Design review of the part built by this model. Coordinates are the model's own, in mm. A direction names the side the tool comes from. Round coordinates to 2 decimals unless told otherwise and drop trailing zeros. Order: outer loops, then holes, each group sorted by start corner. A loop starts at its lowest first (then second) coordinate and runs counter-clockwise, first axis right, second up. Notation, with made-up numbers: M 42.5,-19 L 63.5,-19 A19 cw 63.5,-9 Z; hole C 85,-2.5 d11. An arc over 180 degrees is marked long. Use a Markdown table: item, result. Add a question column.
(1) Take a section at A-A (x = 678.5). Write out the cut boundary in (y, z), then the cut area to 3 significant figures.
(2) The part is to be moulded in two halves that separate along Z. For faces 1 (the face through (832.295, -1.69, 56.85)), 2 (the face through (752, 0, 34)), 3 (the face through (872.457, -1.69, 133.828)), say which applies: released by +Z, released by -Z, zero draft, split by the parting line, or undercut.
(3) For pin 1 (1 mm diameter, centred on y = -1.5, z = 42, fed in from +X); pin 2 (1.7 mm diameter, centred on x = 860.5, y = -1, fed in from -Z); pin 3 (1 mm diameter, centred on y = -1.5, z = 155, fed in from +X); pin 4 (8 mm diameter, centred on x = 598, z = 165, fed in from +Y), all flat-tipped, find the tip position at first contact; note any pin that passes through.
(4) To check wall thickness, follow probe 1 along Z at (x, y) = (849.5, -2.2); probe 2 along Z at (x, y) = (784, -0.8); probe 3 along Z at (x, y) = (637, -1.9). State the ranges of each line that lie inside material, in increasing order. Write a range as from..to.
(5) Take a section at B-B (x = 827). Write out the cut boundary in (y, z), then the cut area to 3 significant figures.
(6) Take a section at C-C (z = 121). Write out the cut boundary in (x, y).
(7) Machinability: for faces 4 (the face through (831.6, -1.7, 141.3)), 5 (the face through (752, -3.429, 34)), which of the approach directions +Z, -Z, +X, -X, +Y, -Y give a long, thin tool a straight path to every point of the face, cutting with its end or side? Answer none if there is none.
(8) Take a section at D-D (z = 78). Write out the cut boundary in (x, y), then the cut area to 3 significant figures.
```python
from build123d import *

# Parameters (mm, degrees)
F0_W     = 3.81
F0_H     = 19.05
F1_DEPTH = 3.429


# Not quite as in the source:
# - ends of sketch curves that miss each other by under 0.0002 mm in the source are joined


with BuildPart() as f1:
    # F0 (on Front) → F1 (new body)
    with BuildSketch(Plane.XZ):
        with BuildLine():
            Line((641.7700144, 153.9733014), (749.7200144, 153.9733014))
            Line((749.7200144, 153.9733014), (749.7200144, 157.1483014))
            Line((749.7200144, 157.1483014), (768.7700144, 157.1483014))
            Line((768.7700144, 157.1483014), (768.7700144, 153.9733014))
            Line((768.7700144, 153.9733014), (800.5200144, 153.9733014))
            ThreePointArc((800.5200144, 153.9733014), (831.9509108237, 140.9541978237), (844.9700144, 109.5233014))
            Line((844.9700144, 109.5233014), (844.9700144, 87.9333014))
            ThreePointArc((844.9700144, 87.9333014), (831.9509108237, 56.5024049763), (800.5200144, 43.4833014))
            Line((800.5200144, 43.4833014), (768.7700144, 43.4833014))
            Line((768.7700144, 43.4833014), (768.7700144, 40.3083014))
            Line((768.7700144, 40.3083014), (749.7200144, 40.3083014))
            Line((749.7200144, 40.3083014), (749.7200144, 43.4833014))
            Line((749.7200144, 43.4833014), (641.7700144, 43.4833014))
            Line((641.7700144, 43.4833014), (641.7700144, 40.3083014))
            Line((641.7700144, 40.3083014), (622.7200144, 40.3083014))
            Line((622.7200144, 40.3083014), (622.7200144, 43.4833014))
            Line((622.7200144, 43.4833014), (559.2200144, 43.4833014))
            Line((559.2200144, 43.4833014), (559.2200144, 33.9583014))
            Line((559.2200144, 33.9583014), (623.5700762, 10.5367836))
            ThreePointArc((623.5700762, 10.5367836), (630.9394695232, 8.4681877562), (638.536009535, 7.5302985912))
            Line((638.536009535, 7.5302985912), (814.9544788, -0.844042))
            ThreePointArc((814.9544788, -0.844042), (848.1989075574, 9.5280670864), (866.95206277, 38.8724395401))
            Line((866.95206277, 38.8724395401), (877.8095982, 87.7019074))
            ThreePointArc((877.8095982, 87.7019074), (879.0206956, 98.7282890028), (877.80959757, 109.7546698599))
            Line((877.80959757, 109.7546698599), (866.9520634, 158.5841634))
            ThreePointArc((866.9520634, 158.5841634), (848.1988981839, 187.9285174732), (814.954479338, 198.3006334659))
            Line((814.954479338, 198.3006334659), (638.5360102, 189.9262902))
            ThreePointArc((638.5360102, 189.9262902), (630.9394701135, 188.9883897624), (623.5700733762, 186.9198015582))
            Line((623.5700733762, 186.9198015582), (559.2200144, 163.4983014))
            Line((559.2200144, 163.4983014), (559.2200144, 153.9733014))
            Line((559.2200144, 153.9733014), (622.7200144, 153.9733014))
            Line((622.7200144, 153.9733014), (622.7200144, 157.1483014))
            Line((622.7200144, 157.1483014), (641.7700144, 157.1483014))
            Line((641.7700144, 157.1483014), (641.7700144, 153.9733014))
        make_face()
        with Locations((860.8450144, 98.7283014)):
            Rectangle(F0_W, F0_H, mode=Mode.SUBTRACT)
    extrude(amount=F1_DEPTH)


solid = f1.part
```
Verdict:
| question | item | result |
|---|---|---|
| 1 | outline | M -3.43,5.63 L 0,5.63 L 0,43.48 L -3.43,43.48 Z; M -3.43,153.97 L 0,153.97 L 0,191.82 L -3.43,191.82 Z |
| 1 | area | 260 mm^2 |
| 2 | face 1 | undercut |
| 2 | face 2 | zero draft |
| 2 | face 3 | released by +Z |
| 3 | pin 1 | stops at x = 867.76 |
| 3 | pin 2 | stops at z = 21.75 |
| 3 | pin 3 | stops at x = 867.86 |
| 3 | pin 4 | stops at y = 0 |
| 4 | probe 1 | z = 10.56..186.9 |
| 4 | probe 2 | z = 0.63..43.48, 153.97..196.83 |
| 4 | probe 3 | z = 7.63..40.31, 157.15..189.83 |
| 5 | outline | M -3.43,0.02 L 0,0.02 L 0,52.23 L -3.43,52.23 Z; M -3.43,145.23 L 0,145.23 L 0,197.44 L -3.43,197.44 Z |
| 5 | area | 358 mm^2 |
| 6 | outline | M 843.46,-3.43 L 875.31,-3.43 L 875.31,0 L 843.46,0 Z |
| 7 | face 4 | -X, +Y, -Y |
| 7 | face 5 | +Z, -Z, +X, -X, -Y |
| 8 | outline | M 843.85,-3.43 L 875.65,-3.43 L 875.65,0 L 843.85,0 Z |
| 8 | area | 109 mm^2 |
